```python
from build123d import *

# Parameters (mm, degrees)
F1_DEPTH = 13
F3_REACH = 70.401
F5_REACH = 197.0178690716
F7_DEPTH = 14.5
F8_W     = 6.5
F8_H     = 7
F9_DEPTH = 2


with BuildPart() as f1:
    # F0 (on Top) → F1 (new body)
    with BuildSketch(Plane.XY):
        Polygon((-43.3400757611, 0), (0, 0), (0, 45.5), (-22.9823845586, 46.4), (-22.9823845586, 23), (-150.9823845586, 23), (-173, 0), align=None)
    extrude(amount=-F1_DEPTH)

    f3_end = Plane(origin=(-11.4911922793, 45.95, -6.5), x_dir=(0.9992341112, -0.0391304348, 0), z_dir=(0.0391304348, 0.9992341112, 0))
    # F2 (on face) → F3 (join, up to a plane its end follows)
    with BuildSketch(Plane.XZ):
        Polygon((-20.9823845586, -13), (-22.9823845586, -13), (0, -19.9144775652), (0, -13), align=None)
    f3_long = extrude(amount=-F3_REACH, mode=Mode.PRIVATE)
    add(split(f3_long, bisect_by=f3_end, keep=Keep.BOTTOM, mode=Mode.PRIVATE))

    f5_end = Plane(origin=(-161.9911922793, 11.5, -6.5), x_dir=(-0.6915115049, -0.7223654467, 0), z_dir=(-0.7223654467, 0.6915115049, 0))
    # F4 (on face) → F5 (join, up to a plane its end follows)
    with BuildSketch(Plane.YZ):
        Polygon((23, -13), (0, -13), (0, -19.9144775652), align=None)
    f5_long = extrude(amount=-F5_REACH, mode=Mode.PRIVATE)
    add(split(f5_long, bisect_by=f5_end, keep=Keep.BOTTOM, mode=Mode.PRIVATE))

    # F6 (on face) → F7 (join)
    with BuildSketch(Plane.XY):
        Polygon((-149.0678093028, 25), (-150.9823845586, 23), (-22.9823845586, 23), (-22.9823845586, 46.4), (-24.9823845586, 46.4783208546), (-24.9823845586, 25), align=None)
    extrude(amount=-F7_DEPTH)

    # F8 (on face) → F9 (cut)
    with BuildSketch(Plane(origin=(0, 25, 0), x_dir=(-1, 0, 0), z_dir=(0, 1, 0))):
        with Locations((143.8178093028, -5.5)):
            Rectangle(F8_W, F8_H)
        with BuildLine():
            ThreePointArc((140.5678093028, -9), (143.8178093028, -12.25), (147.0678093028, -9))
            Line((147.0678093028, -9), (140.5678093028, -9))
        make_face()
        with BuildLine():
            Line((139.0678093028, -9), (132.5678093028, -9))
            ThreePointArc((132.5678093028, -9), (135.8178093028, -12.25), (139.0678093028, -9))
        make_face()
        with Locations((135.8178093028, -5.5)):
            Rectangle(F8_W, F8_H)
        with Locations((127.8178093028, -5.5)):
            Rectangle(F8_W, F8_H)
        with Locations((119.8178093028, -5.5)):
            Rectangle(F8_W, F8_H)
        with Locations((111.8178093028, -5.5)):
            Rectangle(F8_W, F8_H)
        with Locations((103.8178093028, -5.5)):
            Rectangle(F8_W, F8_H)
        with Locations((95.8178093028, -5.5)):
            Rectangle(F8_W, F8_H)
        with Locations((87.8178093028, -5.5)):
            Rectangle(F8_W, F8_H)
        with Locations((79.8178093028, -5.5)):
            Rectangle(F8_W, F8_H)
        with Locations((71.8178093028, -5.5)):
            Rectangle(F8_W, F8_H)
        with Locations((63.8178093028, -5.5)):
            Rectangle(F8_W, F8_H)
        with Locations((55.8178093028, -5.5)):
            Rectangle(F8_W, F8_H)
        with Locations((47.8178093028, -5.5)):
            Rectangle(F8_W, F8_H)
        with Locations((39.8178093028, -5.5)):
            Rectangle(F8_W, F8_H)
        with Locations((31.8178093028, -5.5)):
            Rectangle(F8_W, F8_H)
        with BuildLine():
            Line((35.0678093028, -9), (28.5678093028, -9))
            ThreePointArc((28.5678093028, -9), (31.8178093028, -12.25), (35.0678093028, -9))
        make_face()
        with BuildLine():
            Line((43.0678093028, -9), (36.5678093028, -9))
            ThreePointArc((36.5678093028, -9), (39.8178093028, -12.25), (43.0678093028, -9))
        make_face()
        with BuildLine():
            Line((51.0678093028, -9), (44.5678093028, -9))
            ThreePointArc((44.5678093028, -9), (47.8178093028, -12.25), (51.0678093028, -9))
        make_face()
        with BuildLine():
            Line((59.0678093028, -9), (52.5678093028, -9))
            ThreePointArc((52.5678093028, -9), (55.8178093028, -12.25), (59.0678093028, -9))
        make_face()
        with BuildLine():
            Line((67.0678093028, -9), (60.5678093028, -9))
            ThreePointArc((60.5678093028, -9), (63.8178093028, -12.25), (67.0678093028, -9))
        make_face()
        with BuildLine():
            Line((75.0678093028, -9), (68.5678093028, -9))
            ThreePointArc((68.5678093028, -9), (71.8178093028, -12.25), (75.0678093028, -9))
        make_face()
        with BuildLine():
            Line((83.0678093028, -9), (76.5678093028, -9))
            ThreePointArc((76.5678093028, -9), (79.8178093028, -12.25), (83.0678093028, -9))
        make_face()
        with BuildLine():
            Line((91.0678093028, -9), (84.5678093028, -9))
            ThreePointArc((84.5678093028, -9), (87.8178093028, -12.25), (91.0678093028, -9))
        make_face()
        with BuildLine():
            Line((99.0678093028, -9), (92.5678093028, -9))
            ThreePointArc((92.5678093028, -9), (95.8178093028, -12.25), (99.0678093028, -9))
        make_face()
        with BuildLine():
            Line((107.0678093028, -9), (100.5678093028, -9))
            ThreePointArc((100.5678093028, -9), (103.8178093028, -12.25), (107.0678093028, -9))
        make_face()
        with BuildLine():
            Line((115.0678093028, -9), (108.5678093028, -9))
            ThreePointArc((108.5678093028, -9), (111.8178093028, -12.25), (115.0678093028, -9))
        make_face()
        with BuildLine():
            Line((123.0678093028, -9), (116.5678093028, -9))
            ThreePointArc((116.5678093028, -9), (119.8178093028, -12.25), (123.0678093028, -9))
        make_face()
        with BuildLine():
            Line((131.0678093028, -9), (124.5678093028, -9))
            ThreePointArc((124.5678093028, -9), (127.8178093028, -12.25), (131.0678093028, -9))
        make_face()
    extrude(amount=-F9_DEPTH, mode=Mode.SUBTRACT)


solid = f1.part
```
Input: part model. Units: mm. Frame: model coordinates. Coordinates: 2 decimals unless noted, no trailing zeros. Loops run counter-clockwise (first coordinate to the right, second up) from the corner with the lowest first, then second, coordinate; pieces in that order, holes last. Notation, with made-up numbers: M -32.5,13 L 26.5,13 A22 ccw 26.5,52 Z; hole C 41.25,41 d1. An arc over 180 degrees is marked long. One line per item, written item: value.
(1) Line query: line 1 along Y through (x, z) = (-87, -9.75); line 2 along Z through (x, y) = (-24.5, 44.5); line 3 along X through (y, z) = (36, -6). Output: solid intervals per line, ascending. Write a range as from..to.
Filled in:
line 1: 0..23
line 2: -14.5..0
line 3: -24.98..0
(2) Pin query (flat end, axial travel): pin 1 (2 mm diameter, centred on x = -89.5, z = -6.5, fed in from +Y); pin 2 (1 mm diameter, centred on x = -47.5, y = 24, fed in from -Z); pin 3 (4.5 mm diameter, centred on x = -99.5, z = -4, fed in from +Y); pin 4 (19 mm diameter, centred on x = -84, y = 36.5, fed in from -Z). Return the tip coordinate at first contact, or that it passes through.
Filled in:
pin 1: y = 23
pin 2: z = -14.5
pin 3: y = 25
pin 4: through
(3) Pull-direction query (Z, two-part tool) for faces 1 (the cylindrical face through (-143.75, 24.01, -12.25)), 2 (the flat face through (-11.65, 28.03, -16.41)), 3 (the flat face through (-88, 0, -10)); classes: +Z half, -Z half, draft (parallel to the pull), parting line (faces both ways), or undercut.
Filled in:
face 1: undercut
face 2: -Z half
face 3: draft
(4) Section B-B (x = -41). Output: boundary loops of the cut face in (y, z), and give its area (3 significant figures).
Filled in:
outline: M 0,-19.91 L 23,-13 L 23,-14.5 L 25,-14.5 L 25,-12.03 L 23,-12.03 L 23,-2 L 25,-2 L 25,0 L 0,0 Z
area: 387 mm^2
(5) Section A-A (y = 35). Output: boundary loops of the cut face in (x, z), and give its area (3 significant figures).
Filled in:
outline: M -24.98,-14.5 L -22.98,-14.5 L -22.98,-13 L 0,-19.91 L 0,0 L -24.98,0 Z
area: 407 mm^2
